Source: three-view drawing plus pictorial views. Frame: mm from the lowest corner of the part. Give positions to 0.01 mm unless a question says otherwise; leave off trailing zeros. Write each loop counter-clockwise with the first axis right and the second up, starting at its lowest first coordinate (ties: lowest second). Pieces come first, ordered by that corner, then holes. Notation, with made-up numbers: M 23.5,75 L 68.5,75 A20 cw 68.5,109 Z; hole C 62.25,65.25 d3. An arc over 180 degrees is marked long. One line per question, with ' | ' between items.
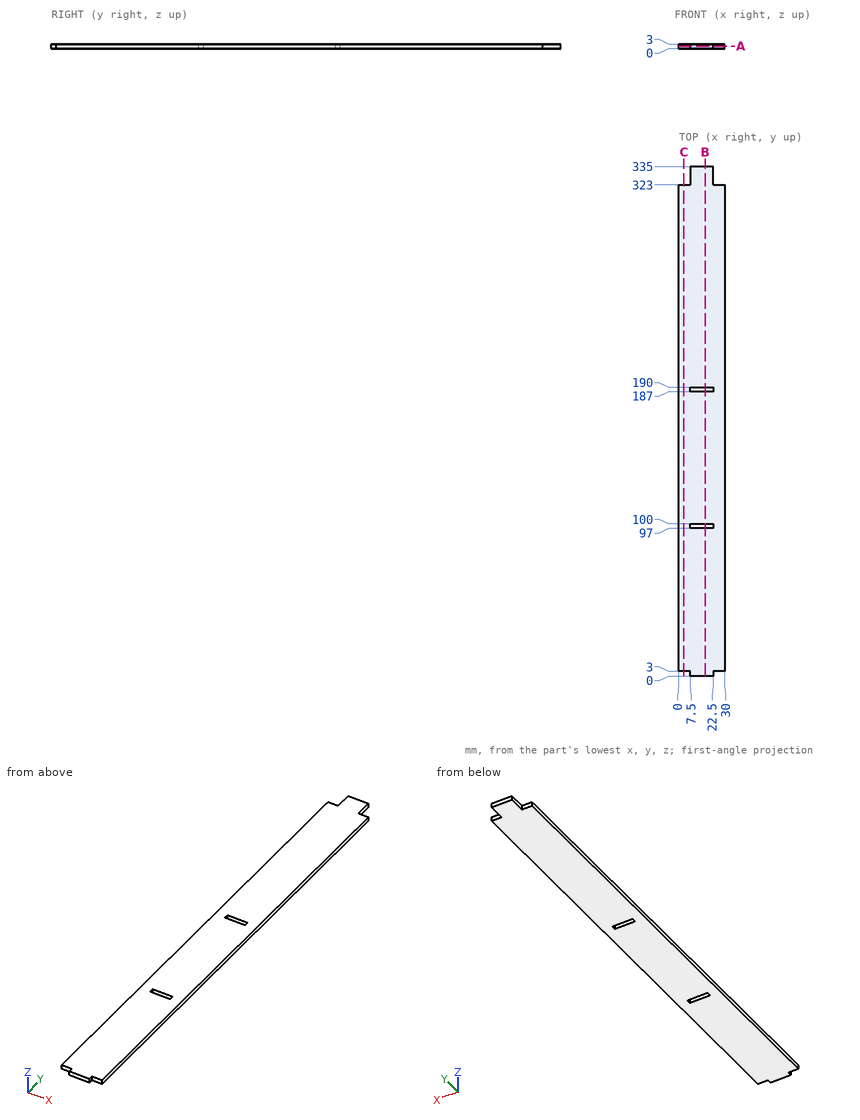
(1) Material intervals for L1, parallel to Y at x = 10, z = 0.5; L2, parallel to Y at x = 4, z = 2.3, sorted ascending. Write a range as [from, to].
Working result:
L1: y = [0, 97], [100, 187], [190, 335] | L2: y = [3, 323]
(2) First-contact query: P1, Ø0.9, axis at x = 25, z = 2, coming from the +Y side; P2, Ø1.5, axis at y = 331, z = 2, coming from the +X side; P3, Ø1.5, axis at x = 26.5, z = 1, coming from the -Y side. Flat tips, straight axial feed; report the tip coordinate or a pass-through.
Working result:
P1: stops at y = 323 | P2: stops at x = 22.5 | P3: stops at y = 3
(3) Cut plane C-C, the plane x = 3.25. Return loops of the section in (y, z).
Working result:
outline: M 3,0 L 323,0 L 323,3 L 3,3 Z
(4) Cut plane A-A, the plane z = 1.55. Return loops of the section in (x, y).
Working result:
outline: M 0,3 L 7.5,3 L 7.5,0 L 22.5,0 L 22.5,3 L 30,3 L 30,323 L 22.5,323 L 22.5,335 L 7.5,335 L 7.5,323 L 0,323 Z; hole M 7.5,97 L 22.5,97 L 22.5,100 L 7.5,100 Z; hole M 7.5,187 L 22.5,187 L 22.5,190 L 7.5,190 Z
(5) Cut plane B-B, the plane x = 17.25. Return loops of the section in (y, z).
Working result:
outline: M 0,0 L 97,0 L 97,3 L 0,3 Z; M 100,0 L 187,0 L 187,3 L 100,3 Z; M 190,0 L 335,0 L 335,3 L 190,3 Z
